from build123d import *

# Parameters (mm, degrees)
BOSS_EXTRUDE1_DEPTH = 60
SKETCH2_W           = 30
SKETCH2_H           = 107.13499281
BOSS_EXTRUDE2_DEPTH = 5
SKETCH3_W           = 80
SKETCH3_H           = 30
BOSS_EXTRUDE3_DEPTH = 5
FILLET2_R           = 10
BOSS_EXTRUDE4_DEPTH = 5
CUT_EXTRUDE2_DEPTH  = 5
SKETCH7_R           = 2.75
CUT_EXTRUDE3_DEPTH  = 178.183520713
SKETCH8_W           = 10
SKETCH8_H           = 6
SKETCH8_W_2         = 6
SKETCH8_H_2         = 10
CUT_EXTRUDE4_DEPTH  = 178.183520713
SKETCH10_R          = 3.585
SKETCH10_W          = 13
SKETCH10_H          = 13
CUT_EXTRUDE5_DEPTH  = 178.183520713
FILLET3_R           = 1.5


with BuildPart() as part:
    # Sketch1 → Boss-Extrude1 (new body)
    with BuildSketch(Plane(origin=(0, 0, 0), x_dir=(1, 0, 0), z_dir=(0, 1, 0))):
        Polygon((0, 0), (0, 100), (3, 100), (3, 3), (83, 3), (83, 100), (86, 100), (86, 0), align=None)
    extrude(amount=BOSS_EXTRUDE1_DEPTH)

    # Sketch2 → Boss-Extrude2 (add)
    with BuildSketch(Plane(origin=(0, 60, 0), x_dir=(1, 0, 0), z_dir=(0, 1, 0))):
        with Locations((98, 66.432503591)):
            Rectangle(SKETCH2_W, SKETCH2_H)
        with Locations((-12, 66.432503591)):
            Rectangle(SKETCH2_W, SKETCH2_H)
    extrude(amount=BOSS_EXTRUDE2_DEPTH)

    # Sketch3 → Boss-Extrude3 (add)
    with BuildSketch(Plane(origin=(0, 65, 0), x_dir=(1, 0, 0), z_dir=(0, 1, 0))):
        with Locations((43, 104.999999996)):
            Rectangle(SKETCH3_W, SKETCH3_H)
    extrude(amount=-BOSS_EXTRUDE3_DEPTH)

    # Fillet2
    fillet2_edges = [part.edges().sort_by_distance(p)[0] for p in [
        (83, 30, -3),
        (3, 30, -3),
        (83, 62.5, -89.999999996),
        (3, 62.5, -89.999999996),
    ]]
    fillet(fillet2_edges, radius=FILLET2_R)
    fillet2_2_edges = [part.edges().sort_by_distance(p)[0] for p in [
        (113, 62.5, -119.999999996),
        (-27, 62.5, -119.999999996),
        (113, 62.5, -12.865007186),
        (-27, 62.5, -12.865007186),
    ]]
    fillet(fillet2_2_edges, radius=FILLET2_R)

    # Sketch5 → Boss-Extrude4 (add)
    with BuildSketch(Plane(origin=(0, 60, 0), x_dir=(1, 0, 0), z_dir=(0, 1, 0))):
        Polygon((0, 12.865007186), (0, 0), (86, 0), (86, 12.865007186), (83, 12.865007186), (83, 3), (3, 3), (3, 12.865007186), align=None)
    extrude(amount=BOSS_EXTRUDE4_DEPTH)

    # Sketch6 → Cut-Extrude2 (cut)
    with BuildSketch(Plane.XY):
        with BuildLine():
            Line((8, 0), (78, 0))
            ThreePointArc((78, 0), (43, 35), (8, 0))
        make_face()
    extrude(amount=-CUT_EXTRUDE2_DEPTH, mode=Mode.SUBTRACT)

    # Sketch7 → Cut-Extrude3 (cut, through all)
    with BuildSketch(Plane(origin=(0, 65, 0), x_dir=(1, 0, 0), z_dir=(0, 1, 0))):
        with Locations(Location((-12, 22.865007186, 0), (0, 0, 270))):
            Circle(SKETCH7_R)
        with Locations(Location((23, 104.999999996, 0), (0, 0, 270))):
            Circle(SKETCH7_R)
        with Locations(Location((98, 22.865007186, 0), (0, 0, 270))):
            Circle(SKETCH7_R)
    extrude(amount=-CUT_EXTRUDE3_DEPTH, mode=Mode.SUBTRACT)

    # Sketch8 → Cut-Extrude4 (cut, through all)
    with BuildSketch(Plane(origin=(0, 65, 0), x_dir=(1, 0, 0), z_dir=(0, 1, 0))):
        with Locations((-12, 52.499999996)):
            Rectangle(SKETCH8_W, SKETCH8_H)
        with Locations((35.581142125, 104.999999996)):
            Rectangle(SKETCH8_W_2, SKETCH8_H_2)
    extrude(amount=-CUT_EXTRUDE4_DEPTH, mode=Mode.SUBTRACT)

    # Sketch10 → Cut-Extrude5 (cut, through all)
    with BuildSketch(Plane(origin=(0, 65, 0), x_dir=(1, 0, 0), z_dir=(0, 1, 0))):
        with Locations(Location((98, 67.865007186, 0), (0, 0, 270))):
            Circle(SKETCH10_R)
        with Locations((98, 47.865007186)):
            Rectangle(SKETCH10_W, SKETCH10_H)
    extrude(amount=-CUT_EXTRUDE5_DEPTH, mode=Mode.SUBTRACT)

    # Fillet3
    fillet3_edges = [part.edges().sort_by_distance(p)[0] for p in [
        (-8.5, 60, -12.865007186),
        (-24.071067812, 60, -15.793939374),
        (-27, 60, -66.432503591),
        (-24.071067812, 60, -117.071067808),
        (43, 60, -119.999999996),
        (110.071067812, 60, -117.071067808),
        (113, 60, -66.432503591),
        (94.5, 60, -12.865007186),
        (110.071067812, 60, -15.793939374),
        (0, 32.5, 0),
        (0, 65, -6.432503593),
        (43, 65, 0),
        (86, 32.5, 0),
        (86, 65, -6.432503593),
        (0, 30, -100),
        (86, 30, -100),
        (43, 35, 0),
    ]]
    fillet(fillet3_edges, radius=FILLET3_R)


solid = part.part
The listing builds one solid part. Answer for the finished solid, in the listing's coordinates (mm). A direction names the side the tool comes from. Give positions to 0.01 mm unless a question says otherwise; leave off trailing zeros. Loops run counter-clockwise (first coordinate to the right, second up) from the corner with the lowest first, then second, coordinate; pieces in that order, holes last. Notation, with made-up numbers: M -7,-23 L 21,-23 A19 cw 21,-19 Z; hole C 78.25,-29 d1. An arc over 180 degrees is marked long. Answer as CSV lines item,"result".
Item 1: Given pin 1 Ø1.5 at (x, y) = (97, 62) entering from +Z (3 decimals); pin 2 Ø4 at (x, z) = (45, -103.5) entering from -Y; pin 3 Ø19.5 at (y, z) = (31, -50) entering from +X, each flat-ended and moving along its own axis, determine where each tip first touches the part or whether it passes through.
Values follow:
pin 1,"stops at z = -12.865"
pin 2,"stops at y = 60"
pin 3,"stops at x = 86"
Item 2: The part is cut by section D-D (x = 98). Give the vertices of the cut face in (y, z) (3 decimals), and give its area (3 significant figures).
Values follow:
outline,"M 60,-118.5 A1.5 ccw 61.5,-120 L 65,-120 L 65,-71.45 L 60,-71.45 Z; M 60,-64.28 L 65,-64.28 L 65,-54.365 L 60,-54.365 Z; M 60,-41.365 L 65,-41.365 L 65,-25.615 L 60,-25.615 Z; M 60,-20.115 L 65,-20.115 L 65,-12.865 L 61.5,-12.865 A1.5 ccw 60,-14.365 Z"
area,"406 mm^2"
Item 3: Straight lines are drawn through the part: line 1 along X through (y, z) = (63.9, -105); line 2 along X through (y, z) = (25, -62); line 3 along X through (y, z) = (61, -105). For each, find the intervals that lie inside material, in ascending order. Write a range as [from, to].
Values follow:
line 1,"x = [-27, 20.25], [25.75, 32.58], [38.58, 113]"
line 2,"x = [0, 3], [83, 86]"
line 3,"x = [-26.91, 20.25], [25.75, 32.58], [38.58, 112.91]"
Item 4: The part is cut by section B-B (z = -105). Give the vertices of the cut face in (x, y), and give its area (3 significant figures).
Values follow:
outline,"M -27,61.5 A1.5 ccw -25.5,60 L 20.25,60 L 20.25,65 L -27,65 Z; M 25.75,60 L 32.58,60 L 32.58,65 L 25.75,65 Z; M 38.58,60 L 111.5,60 A1.5 ccw 113,61.5 L 113,65 L 38.58,65 Z"
area,"642 mm^2"
Item 5: The part is cut by section A-A (x = -12). Give the vertices of the cut face in (y, z) (3 decimals).
Values follow:
outline,"M 60,-118.5 A1.5 ccw 61.5,-120 L 65,-120 L 65,-55.5 L 60,-55.5 Z; M 60,-49.5 L 65,-49.5 L 65,-25.615 L 60,-25.615 Z; M 60,-20.115 L 65,-20.115 L 65,-12.865 L 61.5,-12.865 A1.5 ccw 60,-14.365 Z"
Item 6: The part is cut by section C-C (x = 43). Give the vertices of the cut face in (y, z), and give its area (3 significant figures).
Values follow:
outline,"M 35,-3 L 65,-3 L 65,-1.5 A1.5 ccw 63.5,0 L 36.5,0 A1.5 ccw 35,-1.5 Z; M 60,-118.5 A1.5 ccw 61.5,-120 L 65,-120 L 65,-90 L 60,-90 Z"
area,"239 mm^2"
Item 7: Which of the six approach directions +Z, -Z, +X, -X, +Y, -Y give full straight-line access (tool end or side, diameter ignored) to faces 5 (the flat face through (36, 63, -110)), 6 (the flat face through (5, 60, -5)), 7 (the cylindrical face through (-24.15, 63.27, -116.99))?
Values follow:
face 5,"+Y, -Y"
face 6,"+Y"
face 7,"-Z, -X, +Y, -Y"
Item 8: The mould has two halves that part along X. Classify faces 1 (the flat face through (113, 63, -66)), 2 (the flat face through (91.5, 63, -48)), 3 (the flat face through (42, 65, -101)), 4 (the flat face through (44, 46, -3)): released by +X, released by -X, zero draft, split by the parting line, or undercut.
Values follow:
face 1,"released by +X"
face 2,"undercut"
face 3,"zero draft"
face 4,"undercut"
